Verification items for the finished model (mm, model axes). A direction names the side the tool comes from. Coordinates: 2 decimals unless noted, no trailing zeros. Write each loop counter-clockwise with the first axis right and the second up, starting at its lowest first coordinate (ties: lowest second). Pieces come first, ordered by that corner, then holes. Notation, with made-up numbers: (78.25, 71.5) -> (126.25, 71.5) arc R17 cw to (126.25, 81.5) -> close; hole circle Ø7 at (-24, -15). An arc over 180 degrees is marked (long way). Use CSV: the item, a comma, the result in double quotes.
```python
from build123d import *

# Parameters (mm, degrees)
SKETCH1_R           = 1.6
BOSS_EXTRUDE1_DEPTH = 3
BOSS_EXTRUDE2_DEPTH = 2.1


with BuildPart() as part:
    # Sketch1 → Boss-Extrude1 (new body)
    with BuildSketch(Plane(origin=(0, 0, 0), x_dir=(1, 0, 0), z_dir=(0, 1, 0))):
        with BuildLine():
            Line((-31.5, -29.5), (31.5, -29.5))
            ThreePointArc((31.5, -29.5), (35.742640687, -27.742640687), (37.5, -23.5))
            Line((37.5, -23.5), (37.5, 23.5))
            ThreePointArc((37.5, 23.5), (35.742640687, 27.742640687), (31.5, 29.5))
            Line((31.5, 29.5), (-31.5, 29.5))
            ThreePointArc((-31.5, 29.5), (-35.742640687, 27.742640687), (-37.5, 23.5))
            Line((-37.5, 23.5), (-37.5, -23.5))
            ThreePointArc((-37.5, -23.5), (-35.742640687, -27.742640687), (-31.5, -29.5))
        make_face()
        with Locations(Location((-30, 22, 0), (0, 0, 270))):
            Circle(SKETCH1_R, mode=Mode.SUBTRACT)
        with Locations(Location((30, 22, 0), (0, 0, 270))):
            Circle(SKETCH1_R, mode=Mode.SUBTRACT)
        with Locations(Location((30, -22, 0), (0, 0, 270))):
            Circle(SKETCH1_R, mode=Mode.SUBTRACT)
        with Locations(Location((-30, -22, 0), (0, 0, 270))):
            Circle(SKETCH1_R, mode=Mode.SUBTRACT)
        with BuildLine():
            Line((-27, -22), (-27, -24.6))
            ThreePointArc((-27, -24.6), (-26.853553391, -24.953553391), (-26.5, -25.1))
            Line((-26.5, -25.1), (26.5, -25.1))
            ThreePointArc((26.5, -25.1), (26.853553391, -24.953553391), (27, -24.6))
            Line((27, -24.6), (27, -22))
            ThreePointArc((27, -22), (27.878679656, -19.878679656), (30, -19))
            Line((30, -19), (32.6, -19))
            ThreePointArc((32.6, -19), (32.953553391, -18.853553391), (33.1, -18.5))
            Line((33.1, -18.5), (33.1, 18.5))
            ThreePointArc((33.1, 18.5), (32.953553391, 18.853553391), (32.6, 19))
            Line((32.6, 19), (30, 19))
            ThreePointArc((30, 19), (27.878679656, 19.878679656), (27, 22))
            Line((27, 22), (27, 24.6))
            ThreePointArc((27, 24.6), (26.853553391, 24.953553391), (26.5, 25.1))
            Line((26.5, 25.1), (-26.5, 25.1))
            ThreePointArc((-26.5, 25.1), (-26.853553391, 24.953553391), (-27, 24.6))
            Line((-27, 24.6), (-27, 22))
            ThreePointArc((-27, 22), (-27.878679656, 19.878679656), (-30, 19))
            Line((-30, 19), (-32.6, 19))
            ThreePointArc((-32.6, 19), (-32.953553391, 18.853553391), (-33.1, 18.5))
            Line((-33.1, 18.5), (-33.1, -18.5))
            ThreePointArc((-33.1, -18.5), (-32.953553391, -18.853553391), (-32.6, -19))
            Line((-32.6, -19), (-30, -19))
            ThreePointArc((-30, -19), (-27.878679656, -19.878679656), (-27, -22))
        make_face(mode=Mode.SUBTRACT)
    extrude(amount=BOSS_EXTRUDE1_DEPTH)

    # Sketch2 → Boss-Extrude2 (add)
    with BuildSketch(Plane(origin=(0, 3, 0), x_dir=(1, 0, 0), z_dir=(0, 1, 0))):
        with BuildLine():
            Line((-31.5, -29.5), (31.5, -29.5))
            ThreePointArc((31.5, -29.5), (35.742640687, -27.742640687), (37.5, -23.5))
            Line((37.5, -23.5), (37.5, 23.5))
            ThreePointArc((37.5, 23.5), (35.742640687, 27.742640687), (31.5, 29.5))
            Line((31.5, 29.5), (-31.5, 29.5))
            ThreePointArc((-31.5, 29.5), (-35.742640687, 27.742640687), (-37.5, 23.5))
            Line((-37.5, 23.5), (-37.5, -23.5))
            ThreePointArc((-37.5, -23.5), (-35.742640687, -27.742640687), (-31.5, -29.5))
        make_face()
        with BuildLine():
            Line((-30.1, -25.1), (30.1, -25.1))
            ThreePointArc((30.1, -25.1), (32.221320344, -24.221320344), (33.1, -22.1))
            Line((33.1, -22.1), (33.1, 22.1))
            ThreePointArc((33.1, 22.1), (32.221320344, 24.221320344), (30.1, 25.1))
            Line((30.1, 25.1), (-30.1, 25.1))
            ThreePointArc((-30.1, 25.1), (-32.221320344, 24.221320344), (-33.1, 22.1))
            Line((-33.1, 22.1), (-33.1, -22.1))
            ThreePointArc((-33.1, -22.1), (-32.221320344, -24.221320344), (-30.1, -25.1))
        make_face(mode=Mode.SUBTRACT)
    extrude(amount=BOSS_EXTRUDE2_DEPTH)


solid = part.part
```
1) Set-up check for faces 4 (the flat face through (-31.3, 3, 23.2)), 5 (the cylindrical face through (-27.86, 1.48, -19.9)), 6 (the flat face through (-3, 0, 26)): record each of +Z, -Z, +X, -X, +Y, -Y from which the full face is reachable in a straight line by a thin tool's end or side.
Return value:
face 4,"+Y"
face 5,"+Y, -Y"
face 6,"+Z, -Z, +X, -X, -Y"
2) Gauge pin test, flat ends, axial feed: pin 1 (5.5 mm diameter, centred on x = 28.5, z = -20.5, fed in from +Y); pin 2 (2.5 mm diameter, centred on x = -30, z = 22, fed in from -Y). Record the tip position at first contact, or that the pin passes through.
Return value:
pin 1,"y = 3"
pin 2,"through"
3) Cross-section at A-A (x = 15). Record the boundary of the cut face in (y, z).
Return value:
outline,"(0, -29.5) -> (5.1, -29.5) -> (5.1, -25.1) -> (0, -25.1) -> close; (0, 25.1) -> (5.1, 25.1) -> (5.1, 29.5) -> (0, 29.5) -> close"
4) Scan lines: L1, parallel to X at y = 0.85, z = -22; L2, parallel to Z at x = 13, y = 4; L3, parallel to X at y = 2.2, z = 18. Record each from-to range of solid material in increasing order.
Return value:
L1,"-37.5 to -31.6, -28.4 to -27, 27 to 28.4, 31.6 to 37.5"
L2,"-29.5 to -25.1, 25.1 to 29.5"
L3,"-37.5 to -33.1, 33.1 to 37.5"
5) Cross-section at C-C (z = 5). Record the boundary of the cut face in (x, y), plus the area to 3 significant figures.
Return value:
outline,"(-37.5, 0) -> (-33.1, 0) -> (-33.1, 5.1) -> (-37.5, 5.1) -> close; (33.1, 0) -> (37.5, 0) -> (37.5, 5.1) -> (33.1, 5.1) -> close"
area,"44.9 mm2"
6) Cross-section at B-B (y = 4.1). Record the boundary of the cut face in (x, z).
Return value:
outline,"(-37.5, -23.5) arc R6 ccw to (-31.5, -29.5) -> (31.5, -29.5) arc R6 ccw to (37.5, -23.5) -> (37.5, 23.5) arc R6 ccw to (31.5, 29.5) -> (-31.5, 29.5) arc R6 ccw to (-37.5, 23.5) -> close; hole (-33.1, -22.1) arc R3 ccw to (-30.1, -25.1) -> (30.1, -25.1) arc R3 ccw to (33.1, -22.1) -> (33.1, 22.1) arc R3 ccw to (30.1, 25.1) -> (-30.1, 25.1) arc R3 ccw to (-33.1, 22.1) -> close"
7) Mould release check, pull along Z, two halves, no side actions. Record for faces 1 (the flat face through (31, 1, -19)), 2 (the cylindrical face through (35.789, 2.514, -27.696)), 3 (the flat face through (37.5, 3, 0)): released by +Z, released by -Z, zero draft, split by the parting line, or undercut.
Return value:
face 1,"undercut"
face 2,"released by -Z"
face 3,"zero draft"
